Can you work these out from the model? Positions are in its coordinate system, mm. Coordinates: 2 decimals unless noted, no trailing zeros. Order: outer loops, then holes, each group sorted by start corner. A loop starts at its lowest first (then second) coordinate and runs counter-clockwise, first axis right, second up.
```python
from build123d import *

# Parameters (mm, degrees)
SKETCH1_R           = 2.7
BOSS_EXTRUDE1_DEPTH = 13.5


with BuildPart() as part:
    # Sketch1 → Boss-Extrude1 (new body)
    with BuildSketch(Plane(origin=(0, 0, 0), x_dir=(1, 0, 0), z_dir=(0, 1, 0))):
        with BuildLine():
            Line((20, -15), (-20, -15))
            ThreePointArc((-20, -15), (-23.535533906, -13.535533906), (-25, -10))
            Line((-25, -10), (-25, 10))
            ThreePointArc((-25, 10), (-23.535533906, 13.535533906), (-20, 15))
            Line((-20, 15), (20, 15))
            ThreePointArc((20, 15), (23.535533906, 13.535533906), (25, 10))
            Line((25, 10), (25, -10))
            ThreePointArc((25, -10), (23.535533906, -13.535533906), (20, -15))
        make_face()
        with Locations((-19.5, 0)):
            Circle(SKETCH1_R, mode=Mode.SUBTRACT)
        with Locations((19.5, 0)):
            Circle(SKETCH1_R, mode=Mode.SUBTRACT)
    extrude(amount=BOSS_EXTRUDE1_DEPTH)


solid = part.part
```
1. Please list where these lines run through material, in increasing order: probe 1 along X at (y, z) = (8.5, 0); probe 2 along Z at (x, y) = (19.5, 9); probe 3 along X at (y, z) = (9.25, -1.5) (3 decimals).
Completed:
probe 1: x = -25 to -22.2, -16.8 to 16.8, 22.2 to 25
probe 2: z = -15 to -2.7, 2.7 to 15
probe 3: x = -25 to -21.745, -17.255 to 17.255, 21.745 to 25
2. I'm going to push a flat-ended pin straight in: pin 1 (4.5 mm diameter, centred on x = 19.5, z = 0, fed in from +Y). Where does the tip first touch, or does it pass through?
Completed:
pin 1: passes through
3. Imagine slicing it at D-D on x = -21. Please give me the cut outline in (y, z) (3 decimals).
Completed:
outline: (0, -14.899) - (13.5, -14.899) - (13.5, -2.245) - (0, -2.245) - close; (0, 2.245) - (13.5, 2.245) - (13.5, 14.899) - (0, 14.899) - close
4. Imagine slicing it at B-B on x = 19.5. Please give me the cut outline in (y, z), then the cut area to 3 significant figures.
Completed:
outline: (0, -15) - (13.5, -15) - (13.5, -2.7) - (0, -2.7) - close; (0, 2.7) - (13.5, 2.7) - (13.5, 15) - (0, 15) - close
area: 332 mm2
5. Imagine slicing it at C-C on z = 0. Please give me the cut outline in (x, y).
Completed:
outline: (-25, 0) - (-22.2, 0) - (-22.2, 13.5) - (-25, 13.5) - close; (-16.8, 0) - (16.8, 0) - (16.8, 13.5) - (-16.8, 13.5) - close; (22.2, 0) - (25, 0) - (25, 13.5) - (22.2, 13.5) - close
6. Imagine slicing it at A-A on y = 4. Please give me the cut outline in (x, z).
Completed:
outline: (-25, -10) arc R5 ccw to (-20, -15) - (20, -15) arc R5 ccw to (25, -10) - (25, 10) arc R5 ccw to (20, 15) - (-20, 15) arc R5 ccw to (-25, 10) - close; hole circle Ø5.4 at (-19.5, 0); hole circle Ø5.4 at (19.5, 0)
7. Thinking about a two-plate mould opening in Z: for faces 1 (the cylindrical face through (21.994, 6.656, 1.034)), 2 (the cylindrical face through (-23, 7, 14)), 3 (the cylindrical face through (23, 7, -14)), 4 (the cylindrical face through (-17.006, 6.656, 1.034)), which applies, pulls with the +Z half, pulls with the -Z half, needs draft (parallel to the pull), parting line crosses it, or undercut?
Completed:
face 1: undercut
face 2: pulls with the +Z half
face 3: pulls with the -Z half
face 4: undercut
